For this review, take the finished solid that the model builds, in its own axes (mm). Face numbers are marked on the shaded views. A direction names the side the tool comes from. Give positions to 0.01 mm unless a question says otherwise; leave off trailing zeros. Write each loop counter-clockwise with the first axis right and the second up, starting at its lowest first coordinate (ties: lowest second). Pieces come first, ordered by that corner, then holes. Notation, with made-up numbers: (70.25, 61) -> (97.25, 61) arc R33 ccw to (97.25, 94) -> close; hole circle Ø8 at (14, 64). An arc over 180 degrees is marked (long way). Write item = value, one per line.
```python
from build123d import *

# Parameters (mm, degrees)
SKETCH1_W           = 24
SKETCH1_H           = 32.5
SKETCH1_R           = 1
BOSS_EXTRUDE1_DEPTH = 1.7
SKETCH2_W           = 24
SKETCH2_H           = 24
BOSS_EXTRUDE2_DEPTH = 3.5
SKETCH4_W           = 5
SKETCH4_H           = 5
SKETCH4_H_2         = 8
BOSS_EXTRUDE3_DEPTH = 9


with BuildPart() as part:
    # Sketch1 → Boss-Extrude1 (new body)
    with BuildSketch(Plane(origin=(0, 0, 0), x_dir=(1, 0, 0), z_dir=(0, 1, 0))):
        Rectangle(SKETCH1_W, SKETCH1_H)
        with Locations(Location((0, 14.25, 0), (0, 0, 270))):
            Circle(SKETCH1_R, mode=Mode.SUBTRACT)
        with Locations(Location((0, -14.25, 0), (0, 0, 270))):
            Circle(SKETCH1_R, mode=Mode.SUBTRACT)
    extrude(amount=BOSS_EXTRUDE1_DEPTH)

    # Sketch2 → Boss-Extrude2 (add)
    with BuildSketch(Plane(origin=(0, 1.7, 0), x_dir=(1, 0, 0), z_dir=(0, 1, 0))):
        Rectangle(SKETCH2_W, SKETCH2_H)
    extrude(amount=BOSS_EXTRUDE2_DEPTH)

    # Sketch3 → Revolve1 (revolve)
    with BuildSketch(Plane.XY):
        with BuildLine():
            Line((0, 17.2), (0, 5.2))
            Line((0, 5.2), (12, 5.2))
            ThreePointArc((12, 5.2), (8.485281374, 13.685281374), (0, 17.2))
        make_face()
    revolve(axis=Axis((0, 17.2, 0), (0, -1, 0)))

    # Sketch4 → Boss-Extrude3 (add)
    with BuildSketch(Plane.XZ):
        Polygon((7, 16.25), (12, 16.25), (12, -16.25), (4, -16.25), (4, -12.75), (7, -12.75), align=None)
        with Locations((-9.5, 13.75)):
            Rectangle(SKETCH4_W, SKETCH4_H)
        with Locations((-9.5, -13.75)):
            Rectangle(SKETCH4_W, SKETCH4_H)
        with Locations((-9.5, 0)):
            Rectangle(SKETCH4_W, SKETCH4_H_2)
    extrude(amount=BOSS_EXTRUDE3_DEPTH)


solid = part.part
```
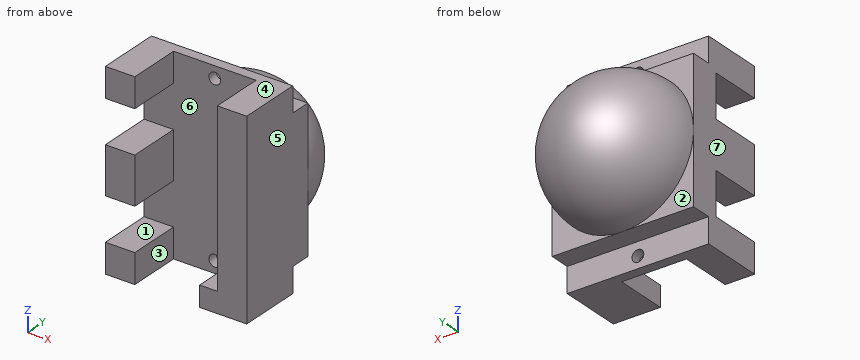
(1) Take a section at B-B (y = -4). Write out the cut boundary in (x, z).
Answers below:
outline = (-12, -16.25) -> (-7, -16.25) -> (-7, -11.25) -> (-12, -11.25) -> close; (-12, -4) -> (-7, -4) -> (-7, 4) -> (-12, 4) -> close; (-12, 11.25) -> (-7, 11.25) -> (-7, 16.25) -> (-12, 16.25) -> close; (4, -16.25) -> (12, -16.25) -> (12, 16.25) -> (7, 16.25) -> (7, -12.75) -> (4, -12.75) -> close
(2) Take a section at A-A (z = -14.25). Write out the cut boundary in (x, y), plus the area to 3 significant figures.
Answers below:
outline = (-12, -9) -> (-7, -9) -> (-7, 0) -> (-1, 0) -> (-1, 1.7) -> (-12, 1.7) -> close; (1, 0) -> (4, 0) -> (4, -9) -> (12, -9) -> (12, 1.7) -> (1, 1.7) -> close
area = 154 mm^2
(3) Take a section at D-D (z = 14.25). Write out the cut boundary in (x, y), plus the area to 3 significant figures.
Answers below:
outline = (-12, -9) -> (-7, -9) -> (-7, 0) -> (-1, 0) -> (-1, 1.7) -> (-12, 1.7) -> close; (1, 0) -> (7, 0) -> (7, -9) -> (12, -9) -> (12, 1.7) -> (1, 1.7) -> close
area = 127 mm^2
(4) To check wall thickness, follow probe 1 along Z at (x, y) = (-10, -3); probe 2 along X at (y, z) = (0.8, -14.25); probe 3 along X at (y, z) = (-4.5, 2). State the ranges of each line that lie inside material, in increasing order.
Answers below:
probe_1 = -16.25 to -11.25, -4 to 4, 11.25 to 16.25
probe_2 = -12 to -1, 1 to 12
probe_3 = -12 to -7, 7 to 12
(5) Tool access review of the marked faces 1, 2 and 3: name each direction out of +Z, -Z, +X, -X, +Y, -Y from which nothing blocks a thin tool from reaching the whole face with its end or side.
Answers below:
face_1 = -X, -Y
face_2 = -Z, -X, +Y
face_3 = +Z, -Z, -Y
(6) For pin 1 (0.9 mm diameter, centred on x = 6, y = -4, fed in from +Z); pin 2 (1 mm diameter, centred on x = -3, y = 3.5, fed in from -Z); pin 3 (1.5 mm diameter, centred on x = 2.5, y = 7, fed in from -Z); pin 4 (1.6 mm diameter, centred on x = 0, z = 14.25, fed in from +Y), all flat-tipped, find the tip position at first contact; note any pin that passes through.
Answers below:
pin_1 = -12.75
pin_2 = -12
pin_3 = -11.77
pin_4 = through
(7) Take a section at C-C (x = 0.5). Count the separate pieces of the cut face and the enclosed holes in it, plus the area to 3 significant figures.
Answers below:
separate_pieces = 3
enclosed_holes = 0
area = 359 mm^2
(8) The part is to be moulded in two halves that separate along X. For the marked faces 4, 5, 6 and 7, say which applies: released by +X, released by -X, zero draft, split by the parting line, or undercut.
Answers below:
face_4 = zero draft
face_5 = released by +X
face_6 = undercut
face_7 = released by -X
